Autodesk Inventor part; units mm, degrees
ref_plane "Work Plane1" through (0, 0, 76.2) normal (0, 0, 1) x (1, 0, 0)
ref_plane "YZ Plane" through (0, 0, 0) normal (1, 0, 0) x (0, 1, 0)
ref_plane "XZ Plane" through (0, 0, 0) normal (0, 1, 0) x (-1, 0, 0)
sketch "Sketch1" plane through (0, 0, 0) normal (0, 0, 1) x (1, 0, 0)
  circle A0 centre (0, 0) radius 25.4
  dimension "d0" = 50.8
extrude "Extrusion1" add sketch "Sketch1" along normal blind 152.4
sketch "Sketch2" plane through (0, 0, 152.4) normal (0, 0, 1) x (1, 0, 0)
  circle A0 centre (0, 0) radius 25.4
  circle A1 centre (0, 0) radius 4.7625
  dimension "d3" = 9.525
extrude "Extrusion2" add sketch "Sketch2" along normal blind 25.4 contours A1
ref_plane "Work Plane1" through (0, 0, 76.2) normal (0, 0, 1) x (1, 0, 0)
sketch "Sketch3" plane through (0, 0, 76.2) normal (0, 0, 1) x (1, 0, 0)
  circle A0 centre (0, 0) radius 25.4
  circle A1 centre (0, 0) radius 24.765
  dimension "d6" = 50.8
  dimension "d7" = 49.53
extrude "Extrusion3" cut sketch "Sketch3" along normal mid plane 2.54
properties part number "SmallMotor_NERDS"
Geometry check sheet. Reference: the model listing, model coordinates, mm. A direction names the side the tool comes from. Give positions to 0.01 mm unless a question says otherwise; leave off trailing zeros. Loops run counter-clockwise (first coordinate to the right, second up) from the corner with the lowest first, then second, coordinate; pieces in that order, holes last. Notation, with made-up numbers: (33.5, 0.25) -> (57.5, 0.25) arc R29 ccw to (57.5, 34.25) -> close; hole circle Ø11 at (80.5, 60.5). An arc over 180 degrees is marked (long way). Answer in a Markdown table with one row per item. Add a question column.
1) Gauge pin test, flat ends, axial feed: P1, Ø5, axis at x = -5.5, z = 79, coming from the -Y side; P2, Ø12, axis at y = -16.5, z = 19.5, coming from the +X side; P3, Ø15, axis at x = 3, y = -6.5, coming from the +Z side; P4, Ø1.5, axis at y = 2, z = 91.5, coming from the -X side. Record the tip position at first contact, or that the pin passes through.
2) Draft check along Z on faces 4 (the face through (-5.506, 24.796, 114.41)), 5 (the face through (0, 0, 177.8)), 6 (the face through (23.62, 7.44, 76.22)), 7 (the face through (5.53, -24.34, 77.47)). Enter one of: pulls with the +Z half, pulls with the -Z half, needs draft (parallel to the pull), parting line crosses it, or undercut.
3) Set-up check for faces 1 (the face through (-3.78, 2.9, 164.92)), 2 (the face through (0, 0, 0)), 3 (the face through (5.53, -24.34, 74.93)): record each of +Z, -Z, +X, -X, +Y, -Y from which the full face is reachable in a straight line by a thin tool's end or side.
4) Cross-section at C-C on z = 146.5. Record the boundary of the cut face in (x, y).
5) Cross-section at D-D on y = 11. Record the boundary of the cut face in (x, z).
6) Material ranges on probe 1 along Z at (x, y) = (18.5, 11); probe 2 along Y at (x, z) = (-1, 99.5); probe 3 along Y at (x, z) = (5.5, 115), recorded low to high. Write a range as from..to.
7) Cross-section at A-A on x = 0. Record the boundary of the cut face in (y, z) (1 decimal), and give its area (3 significant figures).
Outcome:
| question | item | result |
|---|---|---|
| 1 | P1 | stops at y = -25.22 |
| 1 | P2 | stops at x = 23.13 |
| 1 | P3 | stops at z = 177.8 |
| 1 | P4 | stops at x = -25.37 |
| 2 | face 4 | needs draft |
| 2 | face 5 | pulls with the +Z half |
| 2 | face 6 | undercut |
| 2 | face 7 | undercut |
| 3 | face 1 | +Z |
| 3 | face 2 | -Z, +X, -X, +Y, -Y |
| 3 | face 3 | none |
| 4 | outline | circle Ø50.8 at (0, 0) |
| 5 | outline | (-22.89, 0) -> (22.89, 0) -> (22.89, 74.93) -> (22.19, 74.93) -> (22.19, 77.47) -> (22.89, 77.47) -> (22.89, 152.4) -> (-22.89, 152.4) -> (-22.89, 77.47) -> (-22.19, 77.47) -> (-22.19, 74.93) -> (-22.89, 74.93) -> close |
| 6 | probe 1 | z = 0..152.4 |
| 6 | probe 2 | y = -25.38..25.38 |
| 6 | probe 3 | y = -24.8..24.8 |
| 7 | outline | (-25.4, 0) -> (25.4, 0) -> (25.4, 74.9) -> (24.8, 74.9) -> (24.8, 77.5) -> (25.4, 77.5) -> (25.4, 152.4) -> (4.8, 152.4) -> (4.8, 177.8) -> (-4.8, 177.8) -> (-4.8, 152.4) -> (-25.4, 152.4) -> (-25.4, 77.5) -> (-24.8, 77.5) -> (-24.8, 74.9) -> (-25.4, 74.9) -> close |
| 7 | area | 7,980 mm^2 |
